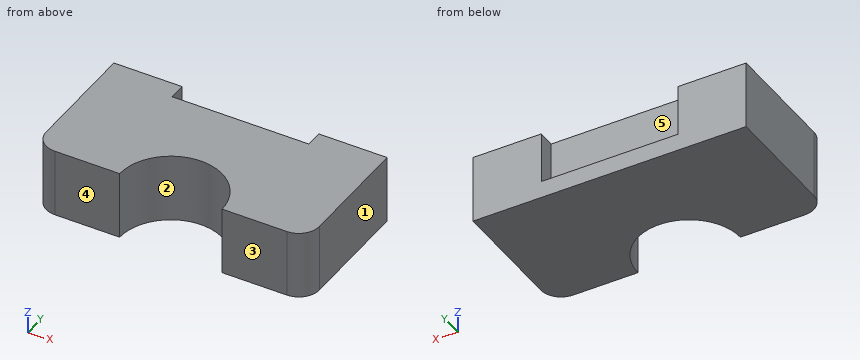
```python
from build123d import *

# Parameters (mm, degrees)
F0_W     = 101.6
F0_H     = 50.8
F1_DEPTH = 25.4
F2_R     = 7.62
F3_W     = 50.8
F3_H     = 6.35
F4_DEPTH = 19.05
F5_R     = 19.05
F6_DEPTH = 25.4


with BuildPart() as f1:
    # F0 (on Top) → F1 (new body)
    with BuildSketch(Plane.XY):
        Rectangle(F0_W, F0_H)
    extrude(amount=F1_DEPTH)

    # F2
    f2_edges = [f1.edges().sort_by_distance(p)[0] for p in [
        (-50.8, -25.4, 12.7),
        (50.8, -25.4, 12.7),
    ]]
    fillet(f2_edges, radius=F2_R)

    # F3 (on face) → F4 (cut)
    with BuildSketch(Plane.XY.offset(25.4)):
        with Locations((0, 22.225)):
            Rectangle(F3_W, F3_H)
    extrude(amount=-F4_DEPTH, mode=Mode.SUBTRACT)

    # F5 (on face) → F6 (cut)
    with BuildSketch(Plane.XY.offset(25.4)):
        with Locations((0, -25.4)):
            Circle(F5_R)
    extrude(amount=-F6_DEPTH, mode=Mode.SUBTRACT)


solid = f1.part
```
Could you check a few things on this model? Use its own coordinates, in mm. Face numbers are marked on the shaded views. A direction names the side the tool comes from. Coordinates: 2 decimals unless noted, no trailing zeros. Loops run counter-clockwise (first coordinate to the right, second up) from the corner with the lowest first, then second, coordinate; pieces in that order, holes last.
1) Will these pins go through, and if not, where does the flat tip stop? pin 1 Ø3 at (x, z) = (10.5, 9) entering from +Y; pin 2 Ø3 at (x, y) = (-10, 23.5) entering from +Z.
Reported:
pin 1: stops at y = 19.05
pin 2: stops at z = 6.35
2) Imagine slicing it at B-B (x = 0). List the corners of the cut face in (y, z) for me.
Reported:
outline: (-6.35, 0) - (25.4, 0) - (25.4, 6.35) - (19.05, 6.35) - (19.05, 25.4) - (-6.35, 25.4) - close
3) Please list where these lines run through material, in increasing order: line 1 along Z through (x, y) = (15, 21.5); line 2 along X through (y, z) = (-21.5, 22.25); line 3 along X through (y, z) = (-22, 13).
Reported:
line 1: z = 0 to 6.35
line 2: x = -49.83 to -18.65, 18.65 to 49.83
line 3: x = -49.52 to -18.74, 18.74 to 49.52
4) Thinking about a two-plate mould opening in X: for the marked faces 1, 2 and 3, which applies, released by +X, released by -X, zero draft, split by the parting line, or undercut?
Reported:
face 1: released by +X
face 2: undercut
face 3: zero draft
5) Imagine slicing it at A-A (y = -21.5). List the corners of the cut face in (x, z) for me, and give its area (3 significant figures).
Reported:
outline: (-49.83, 0) - (-18.65, 0) - (-18.65, 25.4) - (-49.83, 25.4) - close; (18.65, 0) - (49.83, 0) - (49.83, 25.4) - (18.65, 25.4) - close
area: 1,580 mm2
6) Imagine slicing it at D-D (y = -10). List the corners of the cut face in (x, z) for me.
Reported:
outline: (-50.8, 0) - (-11.21, 0) - (-11.21, 25.4) - (-50.8, 25.4) - close; (11.21, 0) - (50.8, 0) - (50.8, 25.4) - (11.21, 25.4) - close
7) Which directions (+Z, -Z, +X, -X, +Y, -Y) give clear straight access to the entire face, cutting with the end or side of a thin tool? Please do the marked faces 4 and 5.
Reported:
face 4: +Z, -Z, +X, -X, -Y
face 5: +Z, +Y
8) Imagine slicing it at C-C (z = 22.5). List the corners of the cut face in (x, y) for me, and give its area (3 significant figures).
Reported:
outline: (-50.8, -17.78) arc R7.62 ccw to (-43.18, -25.4) - (-19.05, -25.4) arc R19.05 cw to (19.05, -25.4) - (43.18, -25.4) arc R7.62 ccw to (50.8, -17.78) - (50.8, 25.4) - (25.4, 25.4) - (25.4, 19.05) - (-25.4, 19.05) - (-25.4, 25.4) - (-50.8, 25.4) - close
area: 4,240 mm2
